from build123d import *

# Parameters (mm, degrees)
EXTRUDE_1_DEPTH          = 2
CUT_EXTRUDE_3_DEPTH      = 26.250159218
CUT_EXTRUDE_3_DEPTH_BACK = 26.250159218
SKETCH_1_3_R             = 2
FILLET_1_R               = 3


with BuildPart() as part:
    # 草图1 → 凸台-拉伸1 (new body)
    with BuildSketch(Plane(origin=(0, 0, 0), x_dir=(0, 0, -1), z_dir=(1, 0, 0))):
        with BuildLine():
            Line((1.479163916, 3.172077255), (-1.479163916, -3.172077255))
            Line((-1.479163916, -3.172077255), (3.19185305, -3.172077255))
            ThreePointArc((3.19185305, -3.172077255), (4.160128527, -1.715613779), (4.5, 0))
            ThreePointArc((4.5, 0), (4.384156276, 1.014482011), (4.042589444, 1.9767323))
            Line((4.042589444, 1.9767323), (1.479163916, 3.172077255))
        make_face()
        with BuildLine():
            Line((1.084261612, -4.36742221), (-1.479163916, -3.172077255))
            Line((-1.479163916, -3.172077255), (-1.479163916, -4.249949895))
            ThreePointArc((-1.479163916, -4.249949895), (-0.206002169, -4.495282317), (1.084261612, -4.36742221))
        make_face()
        with BuildLine():
            Line((3.19185305, -3.172077255), (-1.479163916, -3.172077255))
            Line((-1.479163916, -3.172077255), (1.084261612, -4.36742221))
            ThreePointArc((1.084261612, -4.36742221), (2.220022869, -3.914268573), (3.19185305, -3.172077255))
        make_face()
        with BuildLine():
            Line((-1.479163916, -4.249949895), (-1.479163916, -3.172077255))
            Line((-1.479163916, -3.172077255), (1.479163916, 3.172077255))
            Line((1.479163916, 3.172077255), (4.042589444, 1.9767323))
            ThreePointArc((4.042589444, 1.9767323), (-3.366850219, 2.985685784), (-1.479163916, -4.249949895))
        make_face()
        with BuildLine():
            ThreePointArc((4.5, 0), (4.160128527, -1.715613779), (3.19185305, -3.172077255))
            Line((3.19185305, -3.172077255), (4.520836084, -3.172077255))
            Line((4.520836084, -3.172077255), (4.520836084, -5.969923204))
            Line((4.520836084, -5.969923204), (10.360395407, -8.692954436))
            ThreePointArc((10.360395407, -8.692954436), (9.969385657, -4.648800879), (13.318723239, -2.348799927))
            Line((13.318723239, -2.348799927), (4.042589444, 1.9767323))
            ThreePointArc((4.042589444, 1.9767323), (4.384156276, 1.014482011), (4.5, 0))
        make_face()
        with BuildLine():
            Line((4.520836084, -3.172077255), (3.19185305, -3.172077255))
            ThreePointArc((3.19185305, -3.172077255), (2.220022869, -3.914268573), (1.084261612, -4.36742221))
            Line((1.084261612, -4.36742221), (4.520836084, -5.969923204))
            Line((4.520836084, -5.969923204), (4.520836084, -3.172077255))
        make_face()
        with BuildLine():
            ThreePointArc((1.084261612, -4.36742221), (-0.206002169, -4.495282317), (-1.479163916, -4.249949895))
            Line((-1.479163916, -4.249949895), (-1.479163916, -18))
            Line((-1.479163916, -18), (4.520836084, -18))
            Line((4.520836084, -18), (4.520836084, -5.969923204))
            Line((4.520836084, -5.969923204), (1.084261612, -4.36742221))
        make_face()
        with BuildLine():
            ThreePointArc((17.594616806, -6.339273926), (16.323758221, -3.414930045), (13.318723239, -2.348799927))
            Line((13.318723239, -2.348799927), (15.073780722, -3.167196671))
            Line((15.073780722, -3.167196671), (12.115452889, -9.511351181))
            Line((12.115452889, -9.511351181), (10.360395407, -8.692954436))
            ThreePointArc((10.360395407, -8.692954436), (14.832177795, -10.143014558), (17.594616806, -6.339273926))
        make_face()
        with BuildLine():
            Line((15.073780722, -3.167196671), (13.318723239, -2.348799927))
            ThreePointArc((13.318723239, -2.348799927), (9.969385657, -4.648800879), (10.360395407, -8.692954436))
            Line((10.360395407, -8.692954436), (12.115452889, -9.511351181))
            Line((12.115452889, -9.511351181), (15.073780722, -3.167196671))
        make_face()
    extrude(amount=EXTRUDE_1_DEPTH)

    # 草图1<3> → 切除-拉伸3 (cut, two sides: drawn at the far end of the back side and taken through both)
    with BuildSketch(Plane(origin=(0, 0, 0), x_dir=(0, 0, -1), z_dir=(1, 0, 0)).offset(-CUT_EXTRUDE_3_DEPTH_BACK)):
        Circle(SKETCH_1_3_R)
        with Locations((13.594616806, -6.339273926)):
            Circle(SKETCH_1_3_R)
    extrude(amount=CUT_EXTRUDE_3_DEPTH + CUT_EXTRUDE_3_DEPTH_BACK, mode=Mode.SUBTRACT)

    # 圆角1
    fillet_1_edges = [part.edges().sort_by_distance(p)[0] for p in [
        (1, -2.348799927, -13.318723239),
        (1, 1.9767323, -4.042589444),
        (1, -8.692954436, -10.360395407),
        (1, -5.969923204, -4.520836084),
        (1, -4.249949895, 1.479163916),
    ]]
    fillet(fillet_1_edges, radius=FILLET_1_R)


solid = part.part
Could you check a few things on this model? Use its own coordinates, in mm. A direction names the side the tool comes from. Coordinates: 2 decimals unless noted, no trailing zeros. Loops run counter-clockwise (first coordinate to the right, second up) from the corner with the lowest first, then second, coordinate; pieces in that order, holes last.
1. Imagine slicing it at C-C (x = 0.3). Please give me the cut outline in (y, z).
2. I need wall thicknesses on L1, parallel to Y at x = 0.6, z = 0; L2, parallel to Z at x = 1, y = -6.25; L3, parallel to Z at x = 1.15, y = -12. Which ranges of each line are inside material? Lowest first, please.
3. Imagine slicing it at A-A (z = 0). Please give me the cut outline in (x, y), and give its area (3 significant figures).
4. We'd pull the mould along Z, two halves only. Please class faces 1 (the face through (1, -2, 0)), 2 (the face through (2, -7, -4)), 3 (the face through (1.01, -4.69, 1.79)): released by +Z, released by -Z, zero draft, split by the parting line, or undercut.
5. Imagine slicing it at D-D (y = -16.5). Please give me the cut outline in (x, z), and give its area (3 significant figures).
6. Imagine slicing it at B-B (y = 0). Please give me the cut outline in (x, z), and give its area (3 significant figures).
7. For faces 4 (the face through (1, -12, 1.479)), 5 (the face through (1.01, -2.26, -13.26)), 6 (the face through (1, -8.2, -9.3)), 7 (the face through (1, -14, -4.521)), which set-ups out of +Z, -Z, +X, -X, +Y, -Y let a thin tool reach every point of the face, with its end or its side?
8. For P1, Ø1, axis at x = 1.5, y = -14, coming from the +Z side; P2, Ø10, axis at y = -7.5, z = -13.5, coming from the +X side, each with a flat end and sliding along its axis, tell me the tip position at first contact or that it passes through.
Computed values:
1. outline: (-18, -4.52) - (-10.68, -4.52) arc R3 cw to (-7.96, -8.79) - (-8.41, -9.76) arc R3 cw to (-9.08, -10.68) arc R4 ccw (long way) to (-2.35, -13.82) arc R3 cw to (-2.07, -12.72) - (1.59, -4.87) arc R3 cw to (2.59, -3.68) arc R4.5 ccw (long way) to (-3.61, 2.69) arc R3 cw to (-6.02, 1.48) - (-18, 1.48) - close; hole circle Ø4 at (-6.34, -13.59); hole circle Ø4 at (0, 0)
2. L1: y = -18 to -2, 2 to 4.5
2. L2: z = -17.59 to -15.59, -11.6 to 1.48
2. L3: z = -4.52 to 1.48
3. outline: (0, -18) - (2, -18) - (2, -2) - (0, -2) - close; (0, 2) - (2, 2) - (2, 4.5) - (0, 4.5) - close
3. area: 37.0 mm2
4. face 1: undercut
4. face 2: zero draft
4. face 3: released by +Z
5. outline: (0, -4.52) - (2, -4.52) - (2, 1.48) - (0, 1.48) - close
5. area: 12.0 mm2
6. outline: (0, -8.28) - (2, -8.28) - (2, -2) - (0, -2) - close; (0, 2) - (2, 2) - (2, 4.5) - (0, 4.5) - close
6. area: 17.6 mm2
7. face 4: +Z, +X, -X, -Y
7. face 5: -Z, +X, -X, +Y
7. face 6: +X, -X, -Y
7. face 7: -Z, +X, -X, -Y
8. P1: stops at z = 1.48
8. P2: stops at x = 2
